Build history of the part. All positions in model axes, mm. A direction names the side the tool comes from. Give positions to 0.01 mm unless a question says otherwise; leave off trailing zeros. Order: outer loops, then holes, each group sorted by start corner. A loop starts at its lowest first (then second) coordinate and runs counter-clockwise, first axis right, second up. Notation, with made-up numbers: (58, -10) - (85, -10) arc R20 ccw to (85, 28) - close; hole circle Ø6 at (53.5, 65). An arc over 180 degrees is marked (long way). Use a Markdown table: item, result. Add a question column.
(1) Which spindle directions (+Z, -Z, +X, -X, +Y, -Y) get a long thin tool onto all of the face, cutting with end or side? Do faces 1 (the face through (78, -10.5, -7)), 2 (the face through (26.38, 41.55, 1.97)), 3 (the face through (-72.5, 92, -7)). Say none if no direction does.
(2) Flat gauge pins, fed straight in: pin 1 (5.5 mm diameter, centred on x = 27.4, y = 79.5, fed in from +Z); pin 2 (3.5 mm diameter, centred on x = 27.4, y = 43.5, fed in from +Z); pin 3 (12 mm diameter, centred on x = -55, y = 88.5, fed in from -Z). Where does each tip first touch, or does it go through?
(3) Slice it at C-C (x = 57.5). Write the cut outline in (y, z).
(4) Slice it at D-D (y = 25.5). Write the cut outline in (x, z), then the cut area to 3 significant figures.
(5) Slice it at B-B (y = 0). Write the cut outline in (x, z).
(6) Slice it at A-A (z = -8). Write the cut outline in (x, y).
(7) Wall check: line 1 (Y direction, x = -60.1, z = 3.2); line 2 (Y direction, x = 0, z = 1.3); line 3 (Z direction, x = 42, y = 23.5). Give the ranges that are in metal, low to high.
from build123d import *

# Parameters (mm, degrees)
SKETCH1_W           = 165
SKETCH1_H           = 133
BOSS_EXTRUDE1_DEPTH = 4
SKETCH2_R           = 2.2
CUT_EXTRUDE1_DEPTH  = 4
SKETCH3_W           = 10
SKETCH3_H           = 20
BOSS_EXTRUDE2_DEPTH = 15
CUT_EXTRUDE2_REACH  = 134.429
SKETCH4_R           = 3.1


with BuildPart() as part:
    # Sketch1 → Boss-Extrude1 (new body)
    with BuildSketch(Plane.XY):
        with Locations((0, 36)):
            Rectangle(SKETCH1_W, SKETCH1_H)
    extrude(amount=BOSS_EXTRUDE1_DEPTH)

    # Sketch2 → Cut-Extrude1 (cut)
    with BuildSketch(Plane(origin=(0, 0, 0), x_dir=(-1, 0, 0), z_dir=(0, 0, -1))):
        with Locations((-27.4, 43.5)):
            Circle(SKETCH2_R)
        with Locations((60.1, 43.5)):
            Circle(SKETCH2_R)
        with Locations((60.1, 79.5)):
            Circle(SKETCH2_R)
        with Locations((-27.4, 79.5)):
            Circle(SKETCH2_R)
        with Locations((57.5, 0)):
            Circle(SKETCH2_R)
        with Locations((-57.5, 0)):
            Circle(SKETCH2_R)
    extrude(amount=-CUT_EXTRUDE1_DEPTH, mode=Mode.SUBTRACT)

    # Sketch3 → Boss-Extrude2 (add)
    with BuildSketch(Plane(origin=(0, 0, 0), x_dir=(-1, 0, 0), z_dir=(0, 0, -1))):
        with Locations((-77.5, -20.5)):
            Rectangle(SKETCH3_W, SKETCH3_H)
        with Locations((-77.5, 92.5)):
            Rectangle(SKETCH3_W, SKETCH3_H)
        with Locations((77.5, -20.5)):
            Rectangle(SKETCH3_W, SKETCH3_H)
        with Locations((77.5, 92.5)):
            Rectangle(SKETCH3_W, SKETCH3_H)
    extrude(amount=BOSS_EXTRUDE2_DEPTH)

    # Sketch4 → Cut-Extrude2 (cut, up to next)
    with BuildSketch(Plane(origin=(0, 0, 0), x_dir=(-1, 0, 0), z_dir=(0, 0, -1)), mode=Mode.PRIVATE) as cut_extrude2_sk1:
        with Locations((-72.5, 25.5)):
            Circle(SKETCH4_R)
    cut_extrude2_tool1 = extrude(cut_extrude2_sk1.sketch, amount=-CUT_EXTRUDE2_REACH, mode=Mode.PRIVATE) & part.part
    # Sketch4 → Cut-Extrude2 (cut, up to next)
    with BuildSketch(Plane(origin=(0, 0, 0), x_dir=(-1, 0, 0), z_dir=(0, 0, -1)), mode=Mode.PRIVATE) as cut_extrude2_sk2:
        with Locations((72.5, 25.5)):
            Circle(SKETCH4_R)
    cut_extrude2_tool2 = extrude(cut_extrude2_sk2.sketch, amount=-CUT_EXTRUDE2_REACH, mode=Mode.PRIVATE) & part.part
    # Sketch4 → Cut-Extrude2 (cut, up to next)
    with BuildSketch(Plane(origin=(0, 0, 0), x_dir=(-1, 0, 0), z_dir=(0, 0, -1)), mode=Mode.PRIVATE) as cut_extrude2_sk3:
        with Locations((0, 25.5)):
            Circle(SKETCH4_R)
    cut_extrude2_tool3 = extrude(cut_extrude2_sk3.sketch, amount=-CUT_EXTRUDE2_REACH, mode=Mode.PRIVATE) & part.part
    add(cut_extrude2_tool1.solids().sort_by_distance((72.5, 25.5, 0))[0], mode=Mode.SUBTRACT)
    add(cut_extrude2_tool2.solids().sort_by_distance((-72.5, 25.5, 0))[0], mode=Mode.SUBTRACT)
    add(cut_extrude2_tool3.solids().sort_by_distance((0, 25.5, 0))[0], mode=Mode.SUBTRACT)


solid = part.part
Solution:
| question | item | result |
|---|---|---|
| 1 | face 1 | -Z, +X, -X |
| 1 | face 2 | +Z, -Z |
| 1 | face 3 | -Z, +Y, -Y |
| 2 | pin 1 | z = 4 |
| 2 | pin 2 | through |
| 2 | pin 3 | z = 0 |
| 3 | outline | (-30.5, 0) - (-2.2, 0) - (-2.2, 4) - (-30.5, 4) - close; (2.2, 0) - (102.5, 0) - (102.5, 4) - (2.2, 4) - close |
| 4 | outline | (-82.5, 0) - (-75.6, 0) - (-75.6, 4) - (-82.5, 4) - close; (-69.4, 0) - (-3.1, 0) - (-3.1, 4) - (-69.4, 4) - close; (3.1, 0) - (69.4, 0) - (69.4, 4) - (3.1, 4) - close; (75.6, 0) - (82.5, 0) - (82.5, 4) - (75.6, 4) - close |
| 4 | area | 586 mm2 |
| 5 | outline | (-82.5, 0) - (-59.7, 0) - (-59.7, 4) - (-82.5, 4) - close; (-55.3, 0) - (55.3, 0) - (55.3, 4) - (-55.3, 4) - close; (59.7, 0) - (82.5, 0) - (82.5, 4) - (59.7, 4) - close |
| 6 | outline | (-82.5, -30.5) - (-72.5, -30.5) - (-72.5, -10.5) - (-82.5, -10.5) - close; (-82.5, 82.5) - (-72.5, 82.5) - (-72.5, 102.5) - (-82.5, 102.5) - close; (72.5, -30.5) - (82.5, -30.5) - (82.5, -10.5) - (72.5, -10.5) - close; (72.5, 82.5) - (82.5, 82.5) - (82.5, 102.5) - (72.5, 102.5) - close |
| 7 | line 1 | -30.5 to 41.3, 45.7 to 77.3, 81.7 to 102.5 |
| 7 | line 2 | -30.5 to 22.4, 28.6 to 102.5 |
| 7 | line 3 | 0 to 4 |
